```python
from build123d import *

# Parameters (mm, degrees)
TALADRO_DE_MARGEN_PARA_M162_D = 17.5


with BuildPart() as part:
    # Croquis1 → Revolución3 (revolve)
    with BuildSketch(Plane(origin=(0, 0, 0), x_dir=(1, 0, 0), z_dir=(0, 1, 0))):
        Polygon((0, 33.721279245), (0, -33.721279245), (14, -33.721279245), (32.980229853, -25.290959433), (14, -16.860639622), (32.980229853, -8.430319811), (14, 0), (32.980229853, 8.430319811), (14, 16.860639622), (32.980229853, 25.290959433), (14, 33.721279245), align=None)
    revolve(axis=Axis((0, 0, -33.721279245), (0, 0, 1)))

    # Taladro de margen para M162 (through all)
    with Locations(Plane.XY.offset(33.721279245)):
        with Locations((0, 0.129582741)):
            Hole(TALADRO_DE_MARGEN_PARA_M162_D / 2)


solid = part.part
```
Here's how the part is built. I have some questions about the finished solid (model axes, mm). A direction names the side the tool comes from. Give positions to 0.01 mm unless a question says otherwise; leave off trailing zeros. Order: outer loops, then holes, each group sorted by start corner. A loop starts at its lowest first (then second) coordinate and runs counter-clockwise, first axis right, second up. Notation, with made-up numbers: (59, 10) - (96, 10) arc R22 cw to (96, 28) - close; hole circle Ø5 at (42, 54). An arc over 180 degrees is marked (long way). Answer as a JSON object with one key per item and string values. Group by question number.
Item 1: Which directions (+Z, -Z, +X, -X, +Y, -Y) give clear straight access to the entire face, cutting with the end or side of a thin tool? Please do faces 1 (the conical face through (14.23, 4.48, 17.27)), 2 (the flat face through (0, -9, -33.721)).
Item 2: For P1, Ø4, axis at x = 5.5, z = -22.5, coming from the -Y side; P2, Ø1.5, axis at y = -22, z = 15.5, coming from the +X side; P3, Ø5, axis at y = 8.5, z = -4, coming from the -X side; P4, Ø6, axis at x = 2.5, z = -22, coming from the +Y side, each with a flat end and sliding along its axis, tell me the tip position at first contact or that it passes through.
Item 3: If we section it at A-A on x = 0: Please give me the cut outline in (y, z), and give its area (3 significant figures).
Item 4: If we section it at B-B on z = 5: Please give me the cut outline in (x, y).
Item 5: If we section it at C-C on y = -15: Give the number of separate pieces and of enclosed holes in the cut face, and give its area (3 significant figures).
Item 6: Please list where these lines run through material, in increasing order: probe 1 along Z at (x, y) = (-7, 21); probe 2 along Z at (x, y) = (-11.5, 16); probe 3 along Y at (x, z) = (-2.5, -15).
Item 7: If we mould it in two halves opening along X, with no side actions, what happens to faces 3 (the conical face through (-3.292, -14.826, 33.194)), 4 (the flat face through (0, -9, 33.721)), 5 (the cylindrical face through (6.944, -5.195, -0.472))? For each: pulls with the +X half, pulls with the -X half, needs draft (parallel to the pull), parting line crosses it, or undercut.
Result set:
{
 "1": {"face 1": "none", "face 2": "-Z, +X, -X, +Y, -Y"},
 "2": {"P1": "y = -30.72", "P2": "through", "P3": "x = -27.39", "P4": "y = 32.23"},
 "3": {"outline": "(-32.98, -25.29) - (-14, -33.72) - (-8.62, -33.72) - (-8.62, 33.72) - (-14, 33.72) - (-32.98, 25.29) - (-14, 16.86) - (-32.98, 8.43) - (-14, 0) - (-32.98, -8.43) - (-14, -16.86) - close; (8.88, -33.72) - (14, -33.72) - (32.98, -25.29) - (14, -16.86) - (32.98, -8.43) - (14, 0) - (32.98, 8.43) - (14, 16.86) - (32.98, 25.29) - (14, 33.72) - (8.88, 33.72) - close", "area": "1,990 mm²"},
 "4": {"outline": "circle Ø50.51 at (0, 0); hole circle Ø17.5 at (0, 0.13)"},
 "5": {"separate pieces": "4", "enclosed holes": "0", "area": "2,300 mm²"},
 "6": {"probe 1": "-30.11 to -20.47, -13.25 to -3.61, 3.61 to 13.25, 20.47 to 30.11", "probe 2": "-31.19 to -19.39, -14.33 to -2.53, 2.53 to 14.33, 19.39 to 31.19", "probe 3": "-18.02 to -8.26, 8.51 to 18.02"},
 "7": {"face 3": "parting line crosses it", "face 4": "needs draft", "face 5": "undercut"}
}
